```python
from build123d import *

# Parameters (mm, degrees)
F4_D     = 4.2
F4_DEPTH = 27.8
F4_TIP   = 1.2618073


# Not quite as in the source:
# - a feature of the source that left no trace in its solid (it failed there, or was rolled back) is left out


with BuildPart() as f1:
    # F0 (on Front) → F1 (revolve)
    with BuildSketch(Plane.XZ):
        Polygon((4.9784, 0), (0, 0), (0, -15.6972), (14.4272, -15.6972), (14.4272, 0), (9.779, 0), (9.779, -5.08), (4.9784, -5.08), align=None)
    revolve(axis=Axis((0, 0, -7.8486), (0, 0, 1)))

    # F4
    with Locations(Plane(origin=(0, 0, -15.6972), x_dir=(1, 0, 0), z_dir=(0, 0, -1))):
        with Locations((0, 0)):
            Hole(F4_D / 2, depth=F4_DEPTH)
            with Locations((0, 0, -(F4_DEPTH + F4_TIP / 2))):  # 118° drill point
                Cone(0, F4_D / 2, F4_TIP, mode=Mode.SUBTRACT)


solid = f1.part
```
The listing builds one solid part. Answer for the finished solid, in the listing's coordinates (mm). A direction names the side the tool comes from. Round coordinates to 2 decimals unless told otherwise and drop trailing zeros. Write each loop counter-clockwise with the first axis right and the second up, starting at its lowest first coordinate (ties: lowest second). Pieces come first, ordered by that corner, then holes. Notation, with made-up numbers: (23, 43.25) -> (75, 43.25) arc R23 ccw to (75, 79.25) -> close; hole circle Ø1 at (41, -16.75). An arc over 180 degrees is marked (long way). Answer as a JSON object with one key per item and string values. Group by question number.
Q1. Which of the six approach directions +Z, -Z, +X, -X, +Y, -Y give full straight-line access (tool end or side, diameter ignored) to faces 1 (the face through (-2.003, -0.631, -7.739)), 2 (the face through (4.749, 1.495, -2.504))?
Q2. Determine the mould class of faces 3 (the face through (-11.45, -8.78, -7.74)), 4 (the face through (4, -4, -5.08)), 5 (the face through (0, -3, -15.697)) for opening direction X: pulls with the +X half, pulls with the -X half, needs draft (parallel to the pull), parting line crosses it, or undercut.
Q3. Section A-A (y = 0) is taken. Write down the section's boundary in (x, z), plus the area to 3 significant figures.
Q4. Straight lines are drawn through the part: line 1 along Y through (x, z) = (0, -1.7); line 2 along Y through (x, z) = (0, -10); line 3 along Z through (x, y) = (5.75, 6.5). For each, find the intervals that lie inside material, in ascending order.
Q5. Each of these flat-tipped pins is pushed along its axis until it touches: pin 1 Ø3 at (x, z) = (-9, -9) entering from -Y; pin 2 Ø1.5 at (x, z) = (-4, -6) entering from -Y; pin 3 Ø1.5 at (y, z) = (-10, -9.5) entering from +X; pin 4 Ø4 at (x, y) = (0, 0) entering from -Z. Where does it stop, or does it pass through?
Q6. Section D-D (x = 5.5) is taken. Write down the section's boundary in (y, z).
Q7. Section B-B (z = -4.5) is taken. Write down the section's boundary in (x, y), plus the area to 3 significant figures.
Check values:
{
 "1": {"face 1": "+Z, -Z", "face 2": "+Z"},
 "2": {"face 3": "parting line crosses it", "face 4": "undercut", "face 5": "needs draft"},
 "3": {"outline": "(-14.43, -15.7) -> (-2.1, -15.7) -> (-2.1, 0) -> (-4.98, 0) -> (-4.98, -5.08) -> (-9.78, -5.08) -> (-9.78, 0) -> (-14.43, 0) -> close; (2.1, -15.7) -> (14.43, -15.7) -> (14.43, 0) -> (9.78, 0) -> (9.78, -5.08) -> (4.98, -5.08) -> (4.98, 0) -> (2.1, 0) -> close", "area": "338 mm^2"},
 "4": {"line 1": "-14.43 to -9.78, -4.98 to -2.1, 2.1 to 4.98, 9.78 to 14.43", "line 2": "-14.43 to -2.1, 2.1 to 14.43", "line 3": "-15.7 to -5.08"},
 "5": {"pin 1": "y = -12.32", "pin 2": "y = -14.06", "pin 3": "x = 11.07", "pin 4": "through"},
 "6": {"outline": "(-13.34, -15.7) -> (13.34, -15.7) -> (13.34, 0) -> (8.09, 0) -> (8.09, -5.08) -> (-8.09, -5.08) -> (-8.09, 0) -> (-13.34, 0) -> close"},
 "7": {"outline": "circle Ø28.85 at (0, 0); circle Ø9.96 at (0, 0); hole circle Ø19.56 at (0, 0); hole circle Ø4.2 at (0, 0)", "area": "417 mm^2"}
}
